Geometry check sheet. Reference: the model listing, model coordinates, mm. A direction names the side the tool comes from. Round coordinates to 2 decimals unless told otherwise and drop trailing zeros. Order: outer loops, then holes, each group sorted by start corner. A loop starts at its lowest first (then second) coordinate and runs counter-clockwise, first axis right, second up. Notation, with made-up numbers: (26.5, 78.5) -> (71.5, 78.5) arc R20 cw to (71.5, 105.5) -> close; hole circle Ø10 at (-34, 32). An arc over 180 degrees is marked (long way). Use a Markdown table: item, result. Add a question column.
Item 1: Material ranges on probe 1 along Y at (x, z) = (-80, 2); probe 2 along Y at (x, z) = (-32, -21); probe 3 along X at (y, z) = (1.5, -3.5), recorded low to high. Write a range as [from, to].
Item 2: Sectioned sample at B-B, the plane z = 2.5. Record the cut outline in (x, y).
Item 3: Sectioned sample at C-C, the plane x = -10. Record the cut outline in (y, z), and give its area (3 significant figures).
Item 4: Mould release check, pull along X, two halves, no side actions. Record for faces 6 (the cylindrical face through (-78.092, 0.601, -0.07)), 7 (the flat face through (-10, -7.5, 10)), 8 (the flat face through (-5, 0, -20)): pulls with the +X half, pulls with the -X half, needs draft (parallel to the pull), parting line crosses it, or undercut.
Item 5: Sectioned sample at D-D, the plane z = 10. Record the cut outline in (x, y).
Item 6: Gauge pin test, flat ends, axial feed: pin 1 Ø4 at (y, z) = (1, 11.5) entering from -X; pin 2 Ø2.5 at (x, y) = (-2, 0) entering from -Z; pin 3 Ø4 at (x, y) = (-78.5, -0.5) entering from -Z. Record the tip position at first contact, or that the pin passes through.
Item 7: Sectioned sample at A-A, the plane y = 0. Record the cut outline in (x, z).
Item 8: Set-up check for faces 1 (the flat face through (-78, -1, 5)), 2 (the flat face through (-5, 0, 8)), 3 (the cylindrical face through (-8, -5, 10)), 4 (the flat face through (-75, 0, -15)), 5 (the flat face through (0, 0, -15)): record each of +Z, -Z, +X, -X, +Y, -Y from which the full face is reachable in a straight line by a thin tool's end or side.
from build123d import *

# Parameters (mm, degrees)
BASE_DEPTH          = 5
BASE_DEPTH_BACK     = 5
ESQUISSE1_R         = 2
ESQUISSE2_W         = 75
ESQUISSE2_H         = 5
BOSS_GRAND_DEPTH    = 10
ESQUISSE3_W         = 75
ESQUISSE3_H         = 5
BOSS_PETIT_DEPTH    = 10
ESQUISSE4_W         = 5
ESQUISSE4_H         = 15
BOSS_BLOQUER_DEPTH  = 5
ESQUISSE5_W         = 5
ESQUISSE5_H         = 15
VIDE_BLOQUER_DEPTH  = 5
ESQUISSE6_W         = 70
ESQUISSE6_H         = 5
BOSS_BAS_DEPTH      = 10
ESQUISSE8_R         = 2
ATTACHE_CORDE_DEPTH = 5


with BuildPart() as part:
    # Esquisse1 → BASE (new, two sides: drawn at the far end of the back side and taken through both)
    with BuildSketch(Plane.XY.offset(-BASE_DEPTH_BACK)):
        with BuildLine():
            Line((-80, 2.5), (0, 2.5))
            Line((0, 2.5), (0, -2.5))
            Line((0, -2.5), (-80, -2.5))
            ThreePointArc((-80, -2.5), (-82.5, 0), (-80, 2.5))
        make_face()
        with Locations((-80, 0)):
            Circle(ESQUISSE1_R, mode=Mode.SUBTRACT)
    extrude(amount=BASE_DEPTH + BASE_DEPTH_BACK)

    # Esquisse2 → BOSS GRAND (add)
    with BuildSketch(Plane.XY.offset(5)):
        with Locations((-37.5, 0)):
            Rectangle(ESQUISSE2_W, ESQUISSE2_H)
    extrude(amount=BOSS_GRAND_DEPTH)

    # Esquisse3 → BOSS PETIT (add)
    with BuildSketch(Plane(origin=(0, 0, -5), x_dir=(-1, 0, 0), z_dir=(0, 0, -1))):
        with Locations((37.5, 0)):
            Rectangle(ESQUISSE3_W, ESQUISSE3_H)
    extrude(amount=BOSS_PETIT_DEPTH)

    # Esquisse4 → BOSS BLOQUER (add)
    with BuildSketch(Plane(origin=(0, 2.5, 0), x_dir=(1, 0, 0), z_dir=(0, 1, 0))):
        with Locations((2.5, 7.5)):
            Rectangle(ESQUISSE4_W, ESQUISSE4_H)
    extrude(amount=-BOSS_BLOQUER_DEPTH)

    # Esquisse5 → VIDE BLOQUER (cut)
    with BuildSketch(Plane(origin=(0, 2.5, 0), x_dir=(1, 0, 0), z_dir=(0, 1, 0))):
        with Locations((-2.5, -7.5)):
            Rectangle(ESQUISSE5_W, ESQUISSE5_H)
    extrude(amount=-VIDE_BLOQUER_DEPTH, mode=Mode.SUBTRACT)

    # Esquisse6 → BOSS BAS (add)
    with BuildSketch(Plane(origin=(0, 0, -15), x_dir=(-1, 0, 0), z_dir=(0, 0, -1))):
        with Locations((40, 0)):
            Rectangle(ESQUISSE6_W, ESQUISSE6_H)
    extrude(amount=BOSS_BAS_DEPTH)

    # Esquisse8 → ATTACHE CORDE (add)
    with BuildSketch(Plane.XZ.offset(2.5)):
        with Locations(Location((-10, 10, 0), (0, 0, 270))):
            Circle(ESQUISSE8_R)
    extrude(amount=ATTACHE_CORDE_DEPTH)


solid = part.part
Found:
| question | item | result |
|---|---|---|
| 1 | probe 1 | y = [-2.5, -2], [2, 2.5] |
| 1 | probe 2 | y = [-2.5, 2.5] |
| 1 | probe 3 | x = [-82, -81.32], [-78.68, 5] |
| 2 | outline | (-80, -2.5) -> (-5, -2.5) -> (-5, 2.5) -> (-80, 2.5) arc R2.5 ccw to start; hole circle Ø4 at (-80, 0) |
| 3 | outline | (-7.5, 8) -> (-2.5, 8) -> (-2.5, -25) -> (2.5, -25) -> (2.5, 15) -> (-2.5, 15) -> (-2.5, 12) -> (-7.5, 12) -> close |
| 3 | area | 220 mm2 |
| 4 | face 6 | undercut |
| 4 | face 7 | needs draft |
| 4 | face 8 | pulls with the +X half |
| 5 | outline | (-75, -2.5) -> (-12, -2.5) -> (-12, -7.5) -> (-8, -7.5) -> (-8, -2.5) -> (-5, -2.5) -> (-5, 2.5) -> (-75, 2.5) -> close |
| 6 | pin 1 | stops at x = -75 |
| 6 | pin 2 | stops at z = -15 |
| 6 | pin 3 | stops at z = -5 |
| 7 | outline | (-82.5, -5) -> (-82, -5) -> (-82, 5) -> (-82.5, 5) -> close; (-78, -5) -> (-75, -5) -> (-75, -25) -> (-5, -25) -> (-5, -15) -> (5, -15) -> (5, 0) -> (-5, 0) -> (-5, 15) -> (-75, 15) -> (-75, 5) -> (-78, 5) -> close |
| 8 | face 1 | +Z, -X, +Y, -Y |
| 8 | face 2 | +Z, +X, +Y, -Y |
| 8 | face 3 | -Y |
| 8 | face 4 | -Z, -X, +Y, -Y |
| 8 | face 5 | -Z, +X, +Y, -Y |
